Part model, mm, in its own coordinate system. A direction names the side the tool comes from. Coordinates: 2 decimals unless noted, no trailing zeros. Order: outer loops, then holes, each group sorted by start corner. A loop starts at its lowest first (then second) coordinate and runs counter-clockwise, first axis right, second up.
1) Wall check: L1, parallel to X at y = -1.9, z = -14.5; L2, parallel to X at y = -22.3, z = 0; L3, parallel to Y at x = -9.5, z = 13.5. Give the ranges that are in metal, low to high.
2) Tool access for faces 4 (the cylindrical face through (17.78, -2.46, 14.77)), 5 (the flat face through (0, -21, 17.5)), 6 (the cylindrical face through (-6.834, -12.395, 1.517)), 7 (the cylindrical face through (-17.99, -21.48, -13.39)), 8 (the cylindrical face through (9.667, 11.549, -1.269)): list every direction of +Z, -Z, +X, -X, +Y, -Y with a clear straight run to the whole face (end or side of a thin tool).
3) Mould opens along Y. For faces 1 (the flat face through (-22, -2, 0)), 2 (the flat face through (0, -20, -8)), 3 (the flat face through (0, 16, -11)) say: +Y half, -Y half, draft (parallel to the pull), parting line (faces both ways), or undercut.
4) Cut at D-D (y = 12.5). List the corners of the cut face in (x, z).
5) Pin check, flat tips, straight feed: pin 1 Ø4 at (x, z) = (-19, 14.5) entering from +Y; pin 2 Ø1 at (x, z) = (-4, 7) entering from +Y; pin 3 Ø6 at (y, z) = (7, -8.5) entering from -X. Stop position of each tip, or through.
6) Cut at A-A (x = 19). List the corners of the cut face in (y, z).
```python
from build123d import *

# Parameters (mm, degrees)
SKETCH1_R           = 15.5
BOSS_EXTRUDE1_DEPTH = 16
SKETCH16_W          = 44
SKETCH16_H          = 35
SKETCH16_R          = 1.25
BOSS_EXTRUDE6_DEPTH = 5
SKETCH17_R          = 9.75
CUT_EXTRUDE5_DEPTH  = 6
SKETCH18_R          = 5
CUT_EXTRUDE7_DEPTH  = 19
FILLET4_R           = 1
FILLET1_R           = 1
FILLET3_R           = 1
SKETCH2_R           = 7
BOSS_EXTRUDE3_DEPTH = 20
SKETCH5_R           = 9.75
CUT_EXTRUDE1_DEPTH  = 8
SKETCH6_R           = 5
CUT_EXTRUDE2_DEPTH  = 30
SKETCH12_W          = 44
SKETCH12_H          = 35
BOSS_EXTRUDE4_DEPTH = 3
SKETCH14_R          = 1.5
CUT_EXTRUDE3_DEPTH  = 3
SKETCH15_R          = 5
CUT_EXTRUDE4_DEPTH  = 3


with BuildPart() as part:
    # Sketch1 → Boss-Extrude1 (new body)
    with BuildSketch(Plane(origin=(0, 0, 0), x_dir=(1, 0, 0), z_dir=(0, 1, 0))):
        with Locations(Location((0, 0, 0), (0, 0, 270))):
            Circle(SKETCH1_R)
    extrude(amount=BOSS_EXTRUDE1_DEPTH)

    # Sketch16 → Boss-Extrude6 (add)
    with BuildSketch(Plane.XZ):
        Rectangle(SKETCH16_W, SKETCH16_H)
        with Locations(Location((-19, 14.5, 0), (0, 0, 270))):
            Circle(SKETCH16_R, mode=Mode.SUBTRACT)
        with Locations(Location((19, 14.5, 0), (0, 0, 270))):
            Circle(SKETCH16_R, mode=Mode.SUBTRACT)
        with Locations(Location((19, -14.5, 0), (0, 0, 270))):
            Circle(SKETCH16_R, mode=Mode.SUBTRACT)
        with Locations(Location((-19, -14.5, 0), (0, 0, 270))):
            Circle(SKETCH16_R, mode=Mode.SUBTRACT)
    extrude(amount=BOSS_EXTRUDE6_DEPTH)

    # Sketch17 → Cut-Extrude5 (cut)
    with BuildSketch(Plane(origin=(0, 16, 0), x_dir=(1, 0, 0), z_dir=(0, 1, 0))):
        with Locations(Location((0, 0, 0), (0, 0, 270))):
            Circle(SKETCH17_R)
    extrude(amount=-CUT_EXTRUDE5_DEPTH, mode=Mode.SUBTRACT)

    # Sketch18 → Cut-Extrude7 (cut)
    with BuildSketch(Plane(origin=(0, 10, 0), x_dir=(1, 0, 0), z_dir=(0, 1, 0))):
        with Locations(Location((0, 0, 0), (0, 0, 270))):
            Circle(SKETCH18_R)
    extrude(amount=-CUT_EXTRUDE7_DEPTH, mode=Mode.SUBTRACT)

    # Fillet4
    fillet4_edges = [part.edges().sort_by_distance(p)[0] for p in [
        (0, 0, -15.5),
    ]]
    fillet(fillet4_edges, radius=FILLET4_R)

    # Fillet1
    fillet1_edges = [part.edges().sort_by_distance(p)[0] for p in [
        (0, 16, -9.75),
    ]]
    fillet(fillet1_edges, radius=FILLET1_R)

    # Fillet3
    fillet3_edges = [part.edges().sort_by_distance(p)[0] for p in [
        (0, 16, -15.5),
    ]]
    fillet(fillet3_edges, radius=FILLET3_R)

    # Sketch2 → Boss-Extrude3 (add)
    with BuildSketch(Plane(origin=(0, 0, 0), x_dir=(-1, 0, 0), z_dir=(0, -1, 0))):
        with Locations(Location((0, 0, 0), (0, 0, 90))):
            Circle(SKETCH2_R)
    extrude(amount=BOSS_EXTRUDE3_DEPTH)

    # Sketch5 → Cut-Extrude1 (cut)
    with BuildSketch(Plane(origin=(0, 16, 0), x_dir=(1, 0, 0), z_dir=(0, 1, 0))):
        with Locations(Location((0, 0, 0), (0, 0, 270))):
            Circle(SKETCH5_R)
    extrude(amount=-CUT_EXTRUDE1_DEPTH, mode=Mode.SUBTRACT)

    # Sketch6 → Cut-Extrude2 (cut)
    with BuildSketch(Plane(origin=(0, 8, 0), x_dir=(1, 0, 0), z_dir=(0, 1, 0))):
        with Locations(Location((0, 0, 0), (0, 0, 270))):
            Circle(SKETCH6_R)
    extrude(amount=-CUT_EXTRUDE2_DEPTH, mode=Mode.SUBTRACT)

    # Sketch12 → Boss-Extrude4 (add)
    with BuildSketch(Plane(origin=(0, -20, 0), x_dir=(-1, 0, 0), z_dir=(0, -1, 0))):
        Rectangle(SKETCH12_W, SKETCH12_H)
    extrude(amount=BOSS_EXTRUDE4_DEPTH)

    # Sketch14 → Cut-Extrude3 (cut)
    with BuildSketch(Plane(origin=(0, -20, 0), x_dir=(-1, 0, 0), z_dir=(0, -1, 0))):
        with Locations(Location((-19, -14.5, 0), (0, 0, 90))):
            Circle(SKETCH14_R)
        with Locations(Location((19, -14.5, 0), (0, 0, 90))):
            Circle(SKETCH14_R)
        with Locations(Location((19, 14.5, 0), (0, 0, 90))):
            Circle(SKETCH14_R)
        with Locations(Location((-19, 14.5, 0), (0, 0, 90))):
            Circle(SKETCH14_R)
    extrude(amount=CUT_EXTRUDE3_DEPTH, mode=Mode.SUBTRACT)

    # Sketch15 → Cut-Extrude4 (cut)
    with BuildSketch(Plane(origin=(0, -20, 0), x_dir=(-1, 0, 0), z_dir=(0, -1, 0))):
        with Locations(Location((0, 0, 0), (0, 0, 270))):
            Circle(SKETCH15_R)
    extrude(amount=CUT_EXTRUDE4_DEPTH, mode=Mode.SUBTRACT)


solid = part.part
```
Geometry check:
1. L1: x = -22 to -20.25, -17.75 to 17.75, 20.25 to 22
1. L2: x = -22 to -5, 5 to 22
1. L3: y = -23 to -20, -5 to 0
2. face 4: +Y, -Y
2. face 5: +Z, +X, -X, +Y, -Y
2. face 6: none
2. face 7: -Y
2. face 8: +Y
3. face 1: draft
3. face 2: undercut
3. face 3: +Y half
4. outline: circle Ø31 at (0, 0); hole circle Ø19.5 at (0, 0)
5. pin 1: stops at y = 0
5. pin 2: stops at y = 8
5. pin 3: stops at x = -14.49
6. outline: (-23, -17.5) - (-20, -17.5) - (-20, -16) - (-23, -16) - close; (-23, -13) - (-20, -13) - (-20, 13) - (-23, 13) - close; (-23, 16) - (-20, 16) - (-20, 17.5) - (-23, 17.5) - close; (-5, -17.5) - (0, -17.5) - (0, -15.75) - (-5, -15.75) - close; (-5, -13.25) - (0, -13.25) - (0, 13.25) - (-5, 13.25) - close; (-5, 15.75) - (0, 15.75) - (0, 17.5) - (-5, 17.5) - close
